```python
from build123d import *

# Parameters (mm, degrees)
SKETCH1_R           = 2.175
SKETCH1_R_2         = 1.675
BOSS_EXTRUDE1_DEPTH = 7
SKETCH2_R           = 4.35
CUT_EXTRUDE1_DEPTH  = 3.4
CHAMFER1_SIZE       = 1
CHAMFER2_SIZE       = 0.5


with BuildPart() as part:
    # Sketch1 → Boss-Extrude1 (new body)
    with BuildSketch(Plane.XY):
        with BuildLine():
            Line((-1.4, 6.85857128), (-11, 4.898979486))
            ThreePointArc((-11, 4.898979486), (-15, 0), (-11, -4.898979486))
            Line((-11, -4.898979486), (-1.4, -6.85857128))
            ThreePointArc((-1.4, -6.85857128), (7, 0), (-1.4, 6.85857128))
        make_face()
        Circle(SKETCH1_R, mode=Mode.SUBTRACT)
        with Locations((-10, 0)):
            Circle(SKETCH1_R_2, mode=Mode.SUBTRACT)
    extrude(amount=BOSS_EXTRUDE1_DEPTH)

    # Sketch2 → Cut-Extrude1 (cut)
    with BuildSketch(Plane(origin=(0, 0, 0), x_dir=(-1, 0, 0), z_dir=(0, 0, -1))):
        Circle(SKETCH2_R)
    extrude(amount=-CUT_EXTRUDE1_DEPTH, mode=Mode.SUBTRACT)

    # Chamfer1
    chamfer1_edges = [part.edges().sort_by_distance(p)[0] for p in [
        (-15, 0, 7),
        (-6.2, -5.878775383, 7),
        (7, 0, 7),
        (-6.2, 5.878775383, 7),
    ]]
    chamfer(chamfer1_edges, length=CHAMFER1_SIZE)

    # Chamfer2
    chamfer2_edges = [part.edges().sort_by_distance(p)[0] for p in [
        (-11.675, 0, 0),
        (4.35, 0, 0),
    ]]
    chamfer(chamfer2_edges, length=CHAMFER2_SIZE)


solid = part.part
```
Here's how the part is built. I have some questions about the finished solid (model axes, mm). A direction names the side the tool comes from. Coordinates: 2 decimals unless noted, no trailing zeros. Loops run counter-clockwise (first coordinate to the right, second up) from the corner with the lowest first, then second, coordinate; pieces in that order, holes last. Notation, with made-up numbers: (51, -6.75) - (57, -6.75) arc R14 cw to (57, 13.25) - close; hole circle Ø6 at (33.25, 25.5). An arc over 180 degrees is marked (long way). Return JSON: item names as keys, results as strings. Group by question number.
Item 1: On a 3-axis mill with a long thin cutter (end or side, diameter ignored), from which of +Z, -Z, +X, -X, +Y, -Y can I reach the whole of each face in a straight line? I mean faces 1 (the face through (-2, -2, 3.4)), 2 (the face through (-6.1, 5.9, 3)). Say none if no direction works.
Item 2: If we section it at A-A on x = 0: Write out the boundary of the cut face in (y, z) (3 decimals), and give its area (3 significant figures).
Item 3: I need wall thicknesses on line 1 (X direction, y = 1, z = 1.5); line 2 (Y direction, x = 0, z = 5.9) (3 decimals); line 3 (X direction, y = -0.75, z = 4.25). Which ranges of each line are inside material? Lowest first, please. Write a range as from..to.
Item 4: If we section it at C-C on x = -10: Write out the boundary of the cut face in (y, z) (3 decimals).
Item 5: Will these pins go through, and if not, where does the flat tip stop? P1, Ø1.5, axis at x = -2, z = 1, coming from the -Y side; P2, Ø5, axis at x = 0, y = 0, coming from the -Z side; P3, Ø4.5, axis at x = -1.5, y = -2, coming from the -Z side.
Item 6: We'd pull the mould along Y, two halves only. Please class faces 3 (the face through (-6.166, -5.368, 6.507)), 4 (the face through (-15, 0, 3)), 5 (the face through (-11.673, 0.074, 3.704)): +Y half, -Y half, draft (parallel to the pull), parting line (faces both ways), or undercut.
Item 7: If we section it at B-B on z = 3: Write out the boundary of the cut face in (x, y) (3 decimals).
Item 8: If we section it at D-D on z = 6.5: Write out the boundary of the cut face in (x, y) (3 decimals).
Calculated:
{
 "1": {"face 1": "-Z", "face 2": "+Z, -Z, -X, +Y"},
 "2": {"outline": "(-7, 0) - (-4.85, 0) - (-4.35, 0.5) - (-4.35, 3.4) - (-2.175, 3.4) - (-2.175, 7) - (-6, 7) - (-7, 6) - close; (2.175, 3.4) - (4.35, 3.4) - (4.35, 0.5) - (4.85, 0) - (7, 0) - (7, 6) - (6, 7) - (2.175, 7) - close", "area": "51.5 mm^2"},
 "3": {"line 1": "x = -14.9..-11.34, -8.66..-4.23, 4.23..6.93", "line 2": "y = -7..-2.175, 2.175..7", "line 3": "x = -14.94..-11.5, -8.5..-2.04, 2.04..6.96"},
 "4": {"outline": "(-5.103, 0) - (-2.175, 0) - (-1.675, 0.5) - (-1.675, 7) - (-4.082, 7) - (-5.103, 6) - close; (1.675, 0.5) - (2.175, 0) - (5.103, 0) - (5.103, 6) - (4.082, 7) - (1.675, 7) - close"},
 "5": {"P1": "stops at y = -6.89", "P2": "stops at z = 3.4", "P3": "stops at z = 0.1"},
 "6": {"face 3": "-Y half", "face 4": "parting line", "face 5": "undercut"},
 "7": {"outline": "(-11, -4.899) - (-1.4, -6.859) arc R7 ccw (long way) to (-1.4, 6.859) - (-11, 4.899) arc R5 ccw to start; hole circle Ø3.35 at (-10, 0); hole circle Ø8.7 at (0, 0)"},
 "8": {"outline": "(-10.9, -4.409) - (-1.3, -6.369) arc R6.5 ccw (long way) to (-1.3, 6.369) - (-10.9, 4.409) arc R4.5 ccw to start; hole circle Ø3.35 at (-10, 0); hole circle Ø4.35 at (0, 0)"}
}
